Source: CAD feature listing. Evaluate the final solid. Frame: model axes, mm. A direction names the side the tool comes from. Give positions to 0.01 mm unless a question says otherwise; leave off trailing zeros. Order: outer loops, then holes, each group sorted by start corner. A loop starts at its lowest first (then second) coordinate and runs counter-clockwise, first axis right, second up. Notation, with made-up numbers: (-35, -28.75) -> (6, -28.75) arc R24 cw to (6, -15.75) -> close; hole circle Ø10 at (-19.75, 58.25). An arc over 180 degrees is marked (long way). Use CSV: the item, a comma, the result in double quotes.
```python
from build123d import *

# Parameters (mm, degrees)
F0_W     = 27
F0_H     = 20
F0_R     = 1.5
F0_R_2   = 3
F1_DEPTH = 3
F0_W_2   = 3
F2_DEPTH = 20
F3_R     = 3.75
F3_R_2   = 1
F4_DEPTH = 3


with BuildPart() as f1:
    # F0 (on Top) → F1 (new body)
    with BuildSketch(Plane.XY):
        with Locations((-3.945278, -0.49793)):
            Rectangle(F0_W, F0_H)
        with Locations((-7.445278, -5.49793)):
            Circle(F0_R, mode=Mode.SUBTRACT)
        with Locations((2.554722, -5.49793)):
            Circle(F0_R, mode=Mode.SUBTRACT)
        with Locations((-7.445278, 4.50207)):
            Circle(F0_R, mode=Mode.SUBTRACT)
        with Locations((-2.445278, -0.49793)):
            Circle(F0_R_2, mode=Mode.SUBTRACT)
        with Locations((2.554722, 4.50207)):
            Circle(F0_R, mode=Mode.SUBTRACT)
    extrude(amount=F1_DEPTH)

    # F0 (on Top) → F2 (join)
    with BuildSketch(Plane.XY):
        with Locations((11.054722, -0.49793)):
            Rectangle(F0_W_2, F0_H)
    extrude(amount=F2_DEPTH)

    # F3 (on face) → F4 (cut)
    with BuildSketch(Plane.YZ.offset(12.554722)):
        with Locations((-0.49793, 12)):
            Circle(F3_R)
        with Locations((-0.49793, 5)):
            Circle(F3_R_2)
        with Locations((-0.49793, -2.5)):
            Circle(F3_R_2)
    extrude(amount=-F4_DEPTH, mode=Mode.SUBTRACT)


solid = f1.part
```
1. Section query B-B on x = -3.75. Return loops of the section in (y, z), plus the area to 3 significant figures.
Answer below:
outline,"(-10.5, 0) -> (-3.2, 0) -> (-3.2, 3) -> (-10.5, 3) -> close; (2.2, 0) -> (9.5, 0) -> (9.5, 3) -> (2.2, 3) -> close"
area,"43.8 mm²"
2. Section query A-A on z = 5. Return loops of the section in (x, y), plus the area to 3 significant figures.
Answer below:
outline,"(9.55, -10.5) -> (12.55, -10.5) -> (12.55, -1.5) -> (9.55, -1.5) -> close; (9.55, 0.5) -> (12.55, 0.5) -> (12.55, 9.5) -> (9.55, 9.5) -> close"
area,"54.0 mm²"
3. Ray query, line 1 along X through (y, z) = (-5.75, 1.75); line 2 along X through (y, z) = (6.5, 4); line 3 along Z through (x, y) = (7.75, 5.75). Return the intervals inside material, ascending.
Answer below:
line 1,"x = -17.45 to -8.92, -5.97 to 1.08, 4.03 to 12.55"
line 2,"x = 9.55 to 12.55"
line 3,"z = 0 to 3"
4. Pin query (flat end, axial travel): P1, Ø4, axis at x = -13.5, y = 6.5, coming from the +Z side; P2, Ø2, axis at y = -2, z = 17.5, coming from the -X side. Return the tip coordinate at first contact, or that it passes through.
Answer below:
P1,"stops at z = 3"
P2,"stops at x = 9.55"
5. Section query C-C on y = 1.25. Return loops of the section in (x, z).
Answer below:
outline,"(-17.45, 0) -> (-4.88, 0) -> (-4.88, 3) -> (-17.45, 3) -> close; (-0.01, 0) -> (12.55, 0) -> (12.55, 8.68) -> (9.55, 8.68) -> (9.55, 3) -> (-0.01, 3) -> close; (9.55, 15.32) -> (12.55, 15.32) -> (12.55, 20) -> (9.55, 20) -> close"
6. Access query for faces 5 (the flat face through (9.555, -1, 8)), 6 (the flat face through (1, 0, 0)). Directions: +Z, -Z, +X, -X, +Y, -Y. A direction counts if a zero-diameter tool reaches every point of the face in a straight line with its end or side. Return the directions, or none.
Answer below:
face 5,"+Z, -X, +Y, -Y"
face 6,"-Z, +X, -X, +Y, -Y"
7. Section query D-D on y = -1. Return loops of the section in (x, z).
Answer below:
outline,"(-17.45, 0) -> (-5.4, 0) -> (-5.4, 3) -> (-17.45, 3) -> close; (0.51, 0) -> (12.55, 0) -> (12.55, 4.14) -> (9.55, 4.14) -> (9.55, 3) -> (0.51, 3) -> close; (9.55, 5.86) -> (12.55, 5.86) -> (12.55, 8.28) -> (9.55, 8.28) -> close; (9.55, 15.72) -> (12.55, 15.72) -> (12.55, 20) -> (9.55, 20) -> close"
8. Mould query, pull axis Y, two halves, no side actions, for faces 1 (the flat face through (3, 9.502, 2)), 2 (the cylindrical face through (2.36, -4.01, 1.48)), 3 (the cylindrical face through (-5.442, -0.366, 1.479)), 4 (the flat face through (-7, 0, 3)). Classes: released by +Y, released by -Y, zero draft, split by the parting line, or undercut.
Answer below:
face 1,"released by +Y"
face 2,"undercut"
face 3,"undercut"
face 4,"zero draft"
